Read the model definition and answer for the solid it produces. Units are mm, in the model's axes. A direction names the side the tool comes from. Coordinates: 2 decimals unless noted, no trailing zeros. Write each loop counter-clockwise with the first axis right and the second up, starting at its lowest first coordinate (ties: lowest second). Pieces come first, ordered by that corner, then holes. Notation, with made-up numbers: (2, -38) -> (51, -38) arc R11 cw to (51, -23) -> close; hole circle Ø7 at (87.25, 53). An arc over 180 degrees is marked (long way). Answer in a Markdown table with one row per item. Add a question column.
Item 1: For a pull along X with two mould halves and no side action, classify faces 1 (the face through (44.053, 47.194, 22.185)), 2 (the face through (-1, 64, -3)), 3 (the face through (91.17, 109.59, -1.48)) as +X half, -X half, draft (parallel to the pull), parting line (faces both ways), or undercut.
Item 2: Section A-A on x = 0 is taken. Write down the section's boundary in (y, z).
Item 3: Section D-D on x = 24.5 is taken. Write down the section's boundary in (y, z), then the cut area to 3 significant figures.
Item 4: Given pin 1 Ø1.5 at (y, z) = (-1, -1.5) entering from +X; pin 2 Ø8 at (y, z) = (-20, 33.5) entering from +X; pin 3 Ø3 at (x, z) = (83, 13.5) entering from +Y, each flat-ended and moving along its own axis, determine where each tip first touches the part or whether it passes through.
Item 5: Section C-C on y = 0 is taken. Write down the section's boundary in (x, z), then the cut area to 3 significant figures.
Item 6: Section B-B on z = 10 is taken. Write down the section's boundary in (x, y).
Item 7: Straight lines are drawn through the part: line 1 (Y direction, x = 49, z = 32); line 2 (X direction, y = 106, z = 26); line 3 (X direction, y = 69.5, z = 24.5). For each, find the intervals that lie inside material, in ascending order. Write a range as from..to.
Item 8: Which of the six approach directions +Z, -Z, +X, -X, +Y, -Y give full straight-line access (tool end or side, diameter ignored) to faces 4 (the face through (77, 108, 45)), 5 (the face through (-1, -7, 0))?
Autodesk Inventor part; units mm, degrees
ref_plane "YZ Plane" through (0, 0, 0) normal (1, 0, 0) x (0, 1, 0)
ref_plane "XZ Plane" through (0, 0, 0) normal (0, 1, 0) x (-1, 0, 0)
ref_plane "XY Plane" through (0, 0, 0) normal (0, 0, 1) x (1, 0, 0)
sketch "Sketch1" plane through (0, 0, 0) normal (0, 0, 1) x (1, 0, 0)
  circle A0 centre (0, 0) radius 49 construction
  line L0 (0, 0) -> (49, 0) construction
  circle A1 centre (49, 84.8705) radius 49 construction
  circle A2 centre (-49, 84.8705) radius 49 construction
  circle A3 centre (0, 169.741) radius 49 construction
  circle A4 centre (-98, 169.741) radius 49 construction
  circle A5 centre (98, 169.741) radius 49 construction
  circle A6 centre (-49, 84.8705) radius 36
  circle A7 centre (-98, 169.741) radius 36 construction
  circle A8 centre (0, 169.741) radius 36 construction
  circle A9 centre (98, 169.741) radius 36 construction
  circle A10 centre (49, 84.8705) radius 36
  circle A11 centre (0, 0) radius 36
  line L1 (0, 0) -> (34.6482, -34.6482) construction
  line L2 (0, 0) -> (49, 0) construction
  line L3 (-183.7192, 220.2111) -> (183.7192, 220.2111) construction
  line L4 (-52.5602, 133.741) -> (45.4398, 133.741) construction
  line L5 (-52.5602, 133.741) -> (-77.2006, 133.741) construction
  line L6 (-52.5602, 133.741) -> (28.6753, 133.741) construction
  line L7 (45.4398, 133.741) -> (133.7957, 133.741) construction
  line L8 (45.4398, 133.741) -> (77.2264, 133.741) construction
  circle A12 centre (-49, 84.8705) radius 38
  circle A13 centre (49, 84.8705) radius 38
  circle A14 centre (0, 0) radius 38
  circle A15 centre (0, 169.741) radius 38 construction
  circle A16 centre (98, 169.741) radius 38 construction
  line L9 (-140.4352, 194.241) -> (-125.4414, 220.2111) construction
  line L10 (-140.4352, 194.241) -> (-154.5803, 169.741) construction
  line L11 (140.4352, 194.241) -> (125.4414, 220.2111) construction
  line L12 (140.4352, 194.241) -> (154.5803, 169.741) construction
  line L13 (0, -49) -> (28.2902, -49) construction
  line L14 (0, -49) -> (-28.2902, -49) construction
  line L15 (0, 207.741) -> (0, -38) construction
  circle A17 centre (-98, 169.741) radius 38 construction
  line L16 (-136, 169.741) -> (136, 169.741) construction
  line L17 (-133.7957, 133.741) -> (-183.7192, 220.2111) construction
  line L18 (133.7957, 133.741) -> (183.7192, 220.2111) construction
  line L19 (-28.2902, -49) -> (-105.4982, 84.7282) construction
  line L20 (28.2902, -49) -> (105.511, 84.7505) construction
  line L21 (-93.178, 106.0673) -> (-77.2006, 133.741) construction
  line L22 (-93.178, 106.0673) -> (-61.2232, 106.0673) construction
  line L23 (-93.178, 106.0673) -> (-105.4982, 84.7282) construction
  line L24 (-77.2006, 133.741) -> (-133.7957, 133.741) construction
  line L25 (-105.4982, 84.7282) -> (-133.7957, 133.741) construction
  line L26 (89.6177, 112.2785) -> (77.2264, 133.741) construction
  line L27 (89.6177, 112.2785) -> (114.4005, 112.2785) construction
  line L28 (89.6177, 112.2785) -> (105.511, 84.7505) construction
  line L29 (77.2264, 133.741) -> (133.7957, 133.741) construction
  line L30 (105.511, 84.7505) -> (133.7957, 133.741) construction
  line L31 (77.2264, 133.741) -> (-77.2006, 133.741) construction
  line L32 (77.2264, 133.741) -> (-77.2006, 133.741)
  line L33 (-105.4982, 84.7282) -> (-77.2006, 133.741)
  line L34 (-105.4982, 84.7282) -> (-28.2902, -49)
  line L35 (28.2902, -49) -> (-28.2902, -49)
  line L36 (28.2902, -49) -> (105.511, 84.7505)
  line L37 (77.2264, 133.741) -> (105.511, 84.7505)
  dimension "d6" = 98
  dimension "d7" = 98
  dimension "d19" = 76
  dimension "d20" = 76
  dimension "d21" = 76
  dimension "d22" = 76
  dimension "d0" = 98
  dimension "d3" = 98
  dimension "d4" = 98
  dimension "d5" = 98
  dimension "d8" = 72
  dimension "d9" = 72
  dimension "d10" = 72
  dimension "d11" = 72
  dimension "d12" = 72
  dimension "d13" = 72
  dimension "d14" = 45
  dimension "d15" = 180
  dimension "d16" = 0
  dimension "d17" = 76
  dimension "d18" = 76
  dimension "d23" = 60
  dimension "d24" = 120
extrude "Extrusion1" add sketch "Sketch1" along normal blind 45 contours A12 | A13 | A14
extrude "Extrusion2" add sketch "Sketch1" against normal blind 3 contours A6 | A10 | A11 | A12 | A13 | A14 | L37 L36 L35 L34 L33 L32
sketch "Sketch2" plane through (-49, 84.8705, 0) normal (0, 0, 1) x (1, 0, 0)
  line L0 (-3, -5.5) -> (3, -5.5)
  line L1 (3, -5.5) -> (3, 5.5)
  line L2 (3, 5.5) -> (-3, 5.5)
  line L3 (-3, 5.5) -> (-3, -5.5)
  line L4 (-3, -5.5) -> (3, 5.5) construction
  line L5 (3, -5.5) -> (-3, 5.5) construction
  line L6 (94.9892, -5.5) -> (100.9892, -5.5)
  line L7 (100.9892, -5.5) -> (100.9892, 5.5)
  line L8 (100.9892, 5.5) -> (94.9892, 5.5)
  line L9 (94.9892, 5.5) -> (94.9892, -5.5)
  line L10 (94.9892, -5.5) -> (100.9892, 5.5) construction
  line L11 (100.9892, -5.5) -> (94.9892, 5.5) construction
  line L12 (46, -90.3705) -> (52, -90.3705)
  line L13 (52, -90.3705) -> (52, -79.3705)
  line L14 (52, -79.3705) -> (46, -79.3705)
  line L15 (46, -79.3705) -> (46, -90.3705)
  line L16 (46, -90.3705) -> (52, -79.3705) construction
  line L17 (52, -90.3705) -> (46, -79.3705) construction
  point P0 (49, -84.8705)
  point P1 (0, 0)
  point P2 (97.9892, 0)
  dimension "d29" = 6
  dimension "d30" = 11
  dimension "d31" = 6
  dimension "d32" = 11
  dimension "d33" = 6
  dimension "d34" = 11
extrude "Extrusion3" cut sketch "Sketch2" against normal blind 3
properties part number "base"
Results below:
| question | item | result |
|---|---|---|
| 1 | face 1 | undercut |
| 1 | face 2 | draft |
| 1 | face 3 | +X half |
| 2 | outline | (-49, -3) -> (-5.5, -3) -> (-5.5, 0) -> (-36, 0) -> (-36, 45) -> (-38, 45) -> (-38, 0) -> (-49, 0) -> close; (5.5, -3) -> (133.74, -3) -> (133.74, 0) -> (38, 0) -> (38, 45) -> (36, 45) -> (36, 0) -> (5.5, 0) -> close |
| 3 | outline | (-49, -3) -> (133.74, -3) -> (133.74, 0) -> (113.92, 0) -> (113.92, 45) -> (111.25, 45) -> (111.25, 0) -> (58.49, 0) -> (58.49, 45) -> (55.82, 45) -> (55.82, 0) -> (29.05, 0) -> (29.05, 45) -> (26.38, 45) -> (26.38, 0) -> (-26.38, 0) -> (-26.38, 45) -> (-29.05, 45) -> (-29.05, 0) -> (-49, 0) -> close |
| 3 | area | 1,030 mm2 |
| 4 | pin 1 | stops at x = 56.44 |
| 4 | pin 2 | stops at x = 34.47 |
| 4 | pin 3 | stops at y = 104.56 |
| 5 | outline | (-56.58, -3) -> (-3, -3) -> (-3, 0) -> (-36, 0) -> (-36, 45) -> (-38, 45) -> (-38, 0) -> (-56.58, 0) -> close; (3, -3) -> (56.58, -3) -> (56.58, 0) -> (38, 0) -> (38, 45) -> (36, 45) -> (36, 0) -> (3, 0) -> close |
| 5 | area | 501 mm2 |
| 6 | outline | circle Ø76 at (-49, 84.87); circle Ø76 at (0, 0); circle Ø76 at (49, 84.87); hole circle Ø72 at (-49, 84.87); hole circle Ø72 at (0, 0); hole circle Ø72 at (49, 84.87) |
| 7 | line 1 | y = 46.87..48.87, 120.87..122.87 |
| 7 | line 2 | x = -80.58..-78.15, -19.85..-17.42, 17.42..19.85, 78.15..80.58 |
| 7 | line 3 | x = -83.75..-81.55, -16.45..-14.25, 14.25..16.45, 81.55..83.75 |
| 8 | face 4 | +Z, +X, -X, +Y, -Y |
| 8 | face 5 | +Z |
